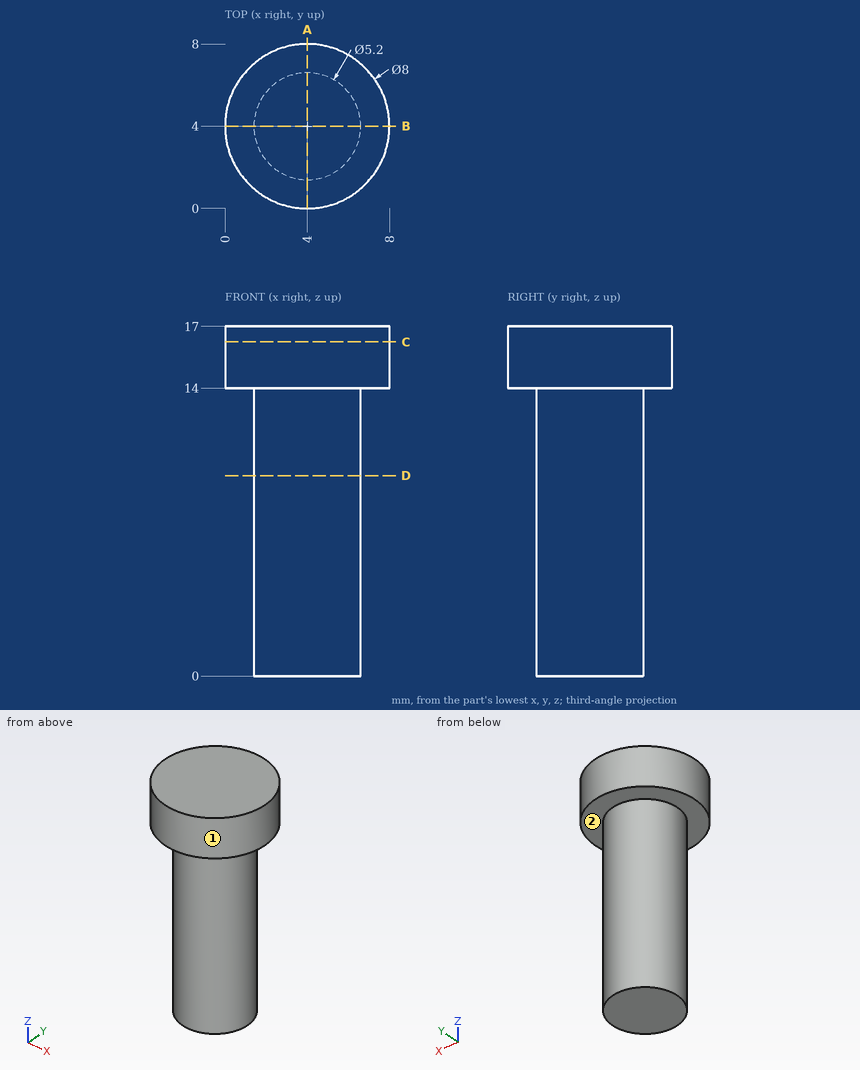
Here's the drawing with two shaded views (mm, measured from the low corner). I have some questions. A direction names the side the tool comes from. Give positions to 0.01 mm unless a question says otherwise; leave off trailing zeros. Order: outer loops, then holes, each group sorted by start corner. A loop starts at its lowest first (then second) coordinate and runs counter-clockwise, first axis right, second up.
Q1. If I drill on line 1 along Z through (x, y) = (6.75, 6.5); line 2 along Y through (x, z) = (4.75, 12); line 3 along Y through (x, z) = (2.75, 0.75), over which ranges is the centre line in solid material (lowest first)?
Q2. Suppose I cut it at A-A, the plane x = 4. Write out the boundary of the cut face in (y, z), and give its area (3 significant figures).
Q3. For the marked faces 1 and 2, which set-ups out of +Z, -Z, +X, -X, +Y, -Y let a thin tool reach every point of the face, with its end or its side?
Q4. Suppose I cut it at C-C, the plane z = 16.25. Write out the boundary of the cut face in (x, y).
Q5. Suppose I cut it at D-D, the plane z = 9.75. Write out the boundary of the cut face in (x, y), and give its area (3 significant figures).
Solution:
1. line 1: z = 14 to 17
1. line 2: y = 1.51 to 6.49
1. line 3: y = 1.72 to 6.28
2. outline: (0, 14) - (1.4, 14) - (1.4, 0) - (6.6, 0) - (6.6, 14) - (8, 14) - (8, 17) - (0, 17) - close
2. area: 96.8 mm2
3. face 1: +Z, -Z
3. face 2: -Z
4. outline: circle Ø8 at (4, 4)
5. outline: circle Ø5.2 at (4, 4)
5. area: 21.2 mm2
